Build history of the part. All positions in model axes, mm. Give positions to 0.01 mm unless a question says otherwise; leave off trailing zeros. Loops run counter-clockwise (first coordinate to the right, second up) from the corner with the lowest first, then second, coordinate; pieces in that order, holes last.
1) Band-saw the part on B-B on x = 48. List the corners of the cut face in (y, z).
2) Wall check: line 1 (X direction, y = -28.5, z = 9); line 2 (Y direction, x = 56, z = 15.5); line 3 (X direction, y = -9.5, z = -13). Give the ranges that are in metal, low to high.
3) Two-plate mould, pull along X, no slides. Class faces 1 (the cylindrical face through (-14.28, -25.04, -0.5)), 2 (the cylindrical face through (-28.57, -25.04, 0.63)), 3 (the flat face through (39, -30.48, 0)), 4 (the cylindrical face through (67.6, -15, 4.3)): +X half, -X half, draft (parallel to the pull), parting line (faces both ways), or undercut.
4) Band-saw the part on A-A on z = 12.5. List the corners of the cut face in (x, y).
5) Band-saw the part on C-C on y = -11.5. State how many separate pieces and enclosed holes the cut face has, then the cut area to 3 significant figures.
6) Flat gauge pins, fed straight in: P1, Ø6, axis at y = -10, z = -5.5, coming from the -X side; P2, Ø1.5, axis at y = -24.5, z = -18, coming from the -X side; P3, Ø4, axis at y = -21, z = -2.5, coming from the -X side. Where does each tip first touch, or does it go through?
```python
from build123d import *
from build123d import SkipClean  # not in build123d's __all__

# Parameters (mm, degrees)
F0_R     = 14.2875
F1_DEPTH = 30.48
F2_DEPTH = 50.8


with BuildPart() as f1:
    # F0 (on Front) → F1 (new body)
    with BuildSketch(Plane.XZ):
        with BuildLine():
            Line((9.5121844836, 26.9452959039), (0, 28.575))
            ThreePointArc((0, 28.575), (-28.575, 0), (0, -28.575))
            Line((0, -28.575), (9.5121844836, -26.9452959039))
            ThreePointArc((9.5121844836, -26.9452959039), (23.3274655355, -16.5033322905), (28.575, 0))
            ThreePointArc((28.575, 0), (23.3274655355, 16.5033322905), (9.5121844836, 26.9452959039))
        make_face()
        with BuildLine():
            ThreePointArc((-13.4703841816, 4.7625), (0, 14.2875), (13.4703841816, 4.7625))
            Line((13.4703841816, 4.7625), (19.05, 4.7625))
            Line((19.05, 4.7625), (19.05, -4.7625))
            Line((19.05, -4.7625), (13.4703841816, -4.7625))
            ThreePointArc((13.4703841816, -4.7625), (0, -14.2875), (-13.4703841816, -4.7625))
            Line((-13.4703841816, -4.7625), (-19.05, -4.7625))
            Line((-19.05, -4.7625), (-19.05, 4.7625))
            Line((-19.05, 4.7625), (-13.4703841816, 4.7625))
        make_face(mode=Mode.SUBTRACT)
        with BuildLine():
            Line((57.1919272622, 18.7764181619), (9.5121844836, 26.9452959039))
            ThreePointArc((9.5121844836, 26.9452959039), (23.3274655355, 16.5033322905), (28.575, 0))
            ThreePointArc((28.575, 0), (23.3274655355, -16.5033322905), (9.5121844836, -26.9452959039))
            Line((9.5121844836, -26.9452959039), (57.1919272622, -18.7764181619))
            ThreePointArc((57.1919272622, -18.7764181619), (34.925, 0), (57.1919272622, 18.7764181619))
        make_face()
        with BuildLine():
            ThreePointArc((73.025, 0), (68.5383952831, 12.2804730295), (57.1919272622, 18.7764181619))
            ThreePointArc((57.1919272622, 18.7764181619), (34.925, 0), (57.1919272622, -18.7764181619))
            ThreePointArc((57.1919272622, -18.7764181619), (68.5383952831, -12.2804730295), (73.025, 0))
        make_face()
        with Locations((53.975, 0)):
            Circle(F0_R, mode=Mode.SUBTRACT)
    extrude(amount=F1_DEPTH)

    # F0 (on Front) → F2 (join)
    with BuildSketch(Plane.XZ):
        with BuildLine():
            Line((9.5121844836, 26.9452959039), (0, 28.575))
            ThreePointArc((0, 28.575), (-28.575, 0), (0, -28.575))
            Line((0, -28.575), (9.5121844836, -26.9452959039))
            ThreePointArc((9.5121844836, -26.9452959039), (23.3274655355, -16.5033322905), (28.575, 0))
            ThreePointArc((28.575, 0), (23.3274655355, 16.5033322905), (9.5121844836, 26.9452959039))
        make_face()
        with BuildLine():
            ThreePointArc((-13.4703841816, 4.7625), (0, 14.2875), (13.4703841816, 4.7625))
            Line((13.4703841816, 4.7625), (19.05, 4.7625))
            Line((19.05, 4.7625), (19.05, -4.7625))
            Line((19.05, -4.7625), (13.4703841816, -4.7625))
            ThreePointArc((13.4703841816, -4.7625), (0, -14.2875), (-13.4703841816, -4.7625))
            Line((-13.4703841816, -4.7625), (-19.05, -4.7625))
            Line((-19.05, -4.7625), (-19.05, 4.7625))
            Line((-19.05, 4.7625), (-13.4703841816, 4.7625))
        make_face(mode=Mode.SUBTRACT)
        with BuildLine():
            ThreePointArc((-13.4703841816, -4.7625), (-14.2875, 0), (-13.4703841816, 4.7625))
            Line((-13.4703841816, 4.7625), (-19.05, 4.7625))
            Line((-19.05, 4.7625), (-19.05, -4.7625))
            Line((-19.05, -4.7625), (-13.4703841816, -4.7625))
        make_face()
        with BuildLine():
            ThreePointArc((13.4703841816, 4.7625), (14.081739421, 2.416044521), (14.2875, 0))
            ThreePointArc((14.2875, 0), (14.081739421, -2.416044521), (13.4703841816, -4.7625))
            Line((13.4703841816, -4.7625), (19.05, -4.7625))
            Line((19.05, -4.7625), (19.05, 4.7625))
            Line((19.05, 4.7625), (13.4703841816, 4.7625))
        make_face()
    with SkipClean():  # cleaning this boolean's faces spoils the solid; the shape is the same uncleaned
        extrude(amount=F2_DEPTH)


solid = f1.part
```
Findings below:
1. outline: (-30.48, -20.35) - (0, -20.35) - (0, -12.98) - (-30.48, -12.98) - close; (-30.48, 12.98) - (0, 12.98) - (0, 20.35) - (-30.48, 20.35) - close
2. line 1: x = -27.12 to -11.1, 11.1 to 42.88, 65.07 to 70.76
2. line 2: y = -30.48 to 0
2. line 3: x = -25.45 to -5.93, 5.93 to 48.05, 59.9 to 67.9
3. face 1: undercut
3. face 2: -X half
3. face 3: draft
3. face 4: undercut
4. outline: (-25.7, -50.8) - (-6.92, -50.8) - (-6.92, 0) - (-25.7, 0) - close; (6.92, -50.8) - (25.7, -50.8) - (25.7, -30.48) - (47.06, -30.48) - (47.06, 0) - (6.92, 0) - close; (60.89, -30.48) - (68.35, -30.48) - (68.35, 0) - (60.89, 0) - close
5. separate pieces: 1
5. enclosed holes: 2
5. area: 3,160 mm2
6. P1: stops at x = -28.47
6. P2: stops at x = -22.78
6. P3: stops at x = -28.57
